Check sheet for the modelled part. Datum: model origin and axes. Units: mm. Coordinates: 2 decimals unless noted, no trailing zeros. Write each loop counter-clockwise with the first axis right and the second up, starting at its lowest first coordinate (ties: lowest second). Pieces come first, ordered by that corner, then holes. Notation, with made-up numbers: (74.25, 66) - (85.25, 66) arc R17 cw to (85.25, 99) - close; hole circle Ø6 at (65.5, 52). An arc over 180 degrees is marked (long way). Answer as CSV lines item,"result". Start each with the question number.
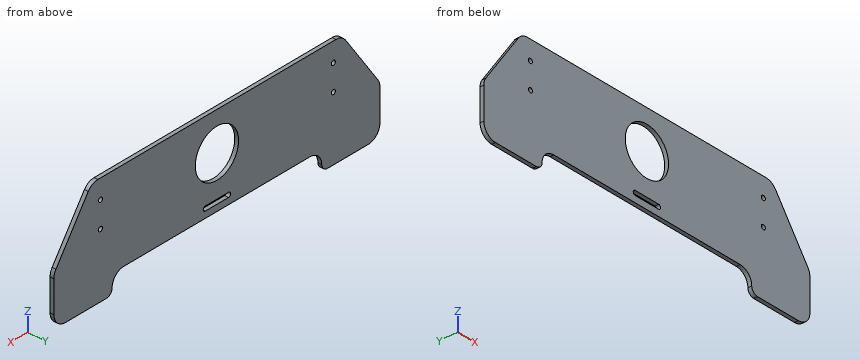
from build123d import *

# Parameters (mm, degrees)
EXTRUDE_1_DEPTH     = 3
SKETCH_4_W          = 287.107775492
SKETCH_4_H          = 19.420897723
CUT_EXTRUDE_2_DEPTH = 18
FILLET_3_R          = 5
FILLET_4_R          = 10
SKETCH_5_R          = 1.75
CUT_EXTRUDE_3_DEPTH = 18
CUT_EXTRUDE_6_DEPTH = 3
SKETCH_9_R          = 18.588109785
CUT_EXTRUDE_7_DEPTH = 10


with BuildPart() as part:
    # 草图1 → 凸台-拉伸1 (new body)
    with BuildSketch(Plane(origin=(0, 0, 0), x_dir=(1, 0, 0), z_dir=(0, 1, 0))):
        with BuildLine():
            Line((-138.235829522, 19.513411872), (-110.492131082, -20.771152042))
            ThreePointArc((-110.492131082, -20.771152042), (-106.908205257, -23.951300285), (-102.25630156, -25.099193643))
            Line((-102.25630156, -25.099193643), (102.25630156, -25.099193643))
            ThreePointArc((102.25630156, -25.099193643), (106.908205257, -23.951300285), (110.492131082, -20.771152042))
            Line((110.492131082, -20.771152042), (138.235829522, 19.513411872))
            ThreePointArc((138.235829522, 19.513411872), (139.548777283, 22.215378286), (140, 25.185370271))
            Line((140, 25.185370271), (140, 65))
            ThreePointArc((140, 65), (137.100120957, 72.000927314), (130.099193643, 74.900806357))
            Line((130.099193643, 74.900806357), (100, 74.900806357))
            ThreePointArc((100, 74.900806357), (92.928932188, 71.971874169), (90, 64.900806357))
            Line((90, 64.900806357), (90, 54.900806357))
            ThreePointArc((90, 54.900806357), (87.071067812, 47.829738545), (80, 44.900806357))
            Line((80, 44.900806357), (-80, 44.900806357))
            ThreePointArc((-80, 44.900806357), (-87.071067812, 47.829738545), (-90, 54.900806357))
            Line((-90, 54.900806357), (-90, 64.900806357))
            ThreePointArc((-90, 64.900806357), (-92.928932188, 71.971874169), (-100, 74.900806357))
            Line((-100, 74.900806357), (-130.099193643, 74.900806357))
            ThreePointArc((-130.099193643, 74.900806357), (-137.100120957, 72.000927314), (-140, 65))
            Line((-140, 65), (-140, 25.185370271))
            ThreePointArc((-140, 25.185370271), (-139.548777283, 22.215378286), (-138.235829522, 19.513411872))
        make_face()
    extrude(amount=EXTRUDE_1_DEPTH)

    # 草图4 → 切除-拉伸2 (cut)
    with BuildSketch(Plane(origin=(0, 3, 0), x_dir=(1, 0, 0), z_dir=(0, 1, 0))):
        with Locations((-3.553887746, 69.611255219)):
            Rectangle(SKETCH_4_W, SKETCH_4_H)
    extrude(amount=-CUT_EXTRUDE_2_DEPTH, mode=Mode.SUBTRACT)

    # 圆角3
    fillet_3_edges = [part.edges().sort_by_distance(p)[0] for p in [
        (-90, 1.5, -59.900806357),
        (90, 1.5, -59.900806357),
    ]]
    fillet(fillet_3_edges, radius=FILLET_3_R - 0.0001)  # a hair under: the kernel refuses the full size

    # 圆角4
    fillet_4_edges = [part.edges().sort_by_distance(p)[0] for p in [
        (140, 1.5, -59.900806357),
        (-140, 1.5, -59.900806357),
    ]]
    fillet(fillet_4_edges, radius=FILLET_4_R)

    # 草图5 → 切除-拉伸3 (cut)
    with BuildSketch(Plane(origin=(0, 3, 0), x_dir=(1, 0, 0), z_dir=(0, 1, 0))):
        with Locations(Location((100, -10.099193643, 0), (0, 0, 270))):
            Circle(SKETCH_5_R)
        with Locations(Location((100, 9.900806357, 0), (0, 0, 270))):
            Circle(SKETCH_5_R)
        with Locations(Location((-100, -10.099193643, 0), (0, 0, 270))):
            Circle(SKETCH_5_R)
        with Locations(Location((-100, 9.900806357, 0), (0, 0, 270))):
            Circle(SKETCH_5_R)
    extrude(amount=-CUT_EXTRUDE_3_DEPTH, mode=Mode.SUBTRACT)

    # 草图8 → 切除-拉伸6 (cut)
    with BuildSketch(Plane(origin=(0, 3, 0), x_dir=(1, 0, 0), z_dir=(0, 1, 0))):
        with BuildLine():
            Line((-10, 39.900806357), (10, 39.900806357))
            ThreePointArc((10, 39.900806357), (11.75, 38.150806357), (10, 36.400806357))
            Line((10, 36.400806357), (-10, 36.400806357))
            ThreePointArc((-10, 36.400806357), (-11.75, 38.150806357), (-10, 39.900806357))
        make_face()
    extrude(amount=-CUT_EXTRUDE_6_DEPTH, mode=Mode.SUBTRACT)

    # 草图9 → 切除-拉伸7 (cut)
    with BuildSketch(Plane.XZ):
        with Locations(Location((0, -4.911890215, 0), (0, 0, 270))):
            Circle(SKETCH_9_R)
    extrude(amount=-CUT_EXTRUDE_7_DEPTH, mode=Mode.SUBTRACT)


solid = part.part
(1) Cross-section at C-C on z = -4. Record the boundary of the cut face in (x, y), plus the area to 3 significant figures.
(2) Go/stop test with flat-tipped pins: P1, Ø5, axis at x = -110.5, z = -48, coming from the -Y side; P2, Ø1.5, axis at y = 0.5, z = 0.5, coming from the -X side; P3, Ø1.5, axis at x = 0, y = 1.5, coming from the -Z side. Record where each tip stops, or that it passes through.
(3) Cross-section at D-D on x = 35.5. Record the boundary of the cut face in (y, z), plus the area to 3 significant figures.
(4) Cross-section at A-A on x = 0. Record the boundary of the cut face in (y, z), plus the area to 3 significant figures.
(5) Material ranges on probe 1 along Z at (x, y) = (100, 1.9); probe 2 along X at (y, z) = (2.3, -38); probe 3 along Z at (x, y) = (36, 1.7), recorded low to high. Write a range as from..to.
(6) Cross-section at B-B on y = 1.15. State how many separate pieces and enclosed holes the cut face has, plus the area to 3 significant figures.
Checked values:
1,outline,"(-127.55, 0) - (-18.57, 0) - (-18.57, 3) - (-127.55, 3) - close; (18.57, 0) - (127.55, 0) - (127.55, 3) - (18.57, 3) - close"
1,area,"654 mm^2"
2,P1,"y = 0"
2,P2,"x = -124.97"
2,P3,"z = -44.9"
3,outline,"(0, -44.9) - (3, -44.9) - (3, 25.1) - (0, 25.1) - close"
3,area,"210 mm^2"
4,outline,"(0, -44.9) - (3, -44.9) - (3, -39.9) - (0, -39.9) - close; (0, -36.4) - (3, -36.4) - (3, -23.5) - (0, -23.5) - close; (0, 13.68) - (3, 13.68) - (3, 25.1) - (0, 25.1) - close"
4,area,"88.0 mm^2"
5,probe 1,"-59.9..-11.65, -8.15..8.35, 11.85..25.1"
5,probe 2,"-140..-11.74, 11.74..140"
5,probe 3,"-44.9..25.1"
6,separate pieces,"1"
6,enclosed holes,"6"
6,area,"18,300 mm^2"
